Design review of the part built by this model. Coordinates are the model's own, in mm. Give positions to 0.01 mm unless a question says otherwise; leave off trailing zeros. Order: outer loops, then holes, each group sorted by start corner. A loop starts at its lowest first (then second) coordinate and runs counter-clockwise, first axis right, second up. Notation, with made-up numbers: (52.5, 15.25) -> (98.5, 15.25) arc R31 ccw to (98.5, 45.25) -> close; hole circle Ø11 at (-31.75, 81.5). An arc over 180 degrees is marked (long way). Return JSON: item names as keys, results as strings.
```python
from build123d import *

# Parameters (mm, degrees)
SKETCH_1_R      = 1.6
EXTRUDE_1_DEPTH = 2
FILLET_1_R      = 2
FILLET_2_R      = 10
SKETCH_2_R      = 2.5
EXTRUDE_2_DEPTH = 5
SKETCH_3_W      = 23
SKETCH_3_H      = 10
EXTRUDE_4_DEPTH = 5


with BuildPart() as part:
    # 草图1 → 凸台-拉伸1 (new body)
    with BuildSketch(Plane(origin=(0, 0, 0), x_dir=(1, 0, 0), z_dir=(0, 1, 0))):
        Polygon((-11.5, 4.501120792), (11.5, 4.501120792), (11.5, 1.918654762), (40, 1.918654762), (56.146384284, 15.918654762), (90, 15.918654762), (90, 29.918654762), (-90, 29.918654762), (-90, 15.918654762), (-56.146384284, 15.918654762), (-40, 1.918654762), (-11.5, 1.918654762), align=None)
        with Locations(Location((17.5, 7.896444982, 0), (0, 0, 270))):
            Circle(SKETCH_1_R, mode=Mode.SUBTRACT)
        with Locations(Location((25, 7.896444982, 0), (0, 0, 270))):
            Circle(SKETCH_1_R, mode=Mode.SUBTRACT)
        with Locations(Location((32.5, 7.896444982, 0), (0, 0, 270))):
            Circle(SKETCH_1_R, mode=Mode.SUBTRACT)
        with Locations(Location((-32.5, 7.896444982, 0), (0, 0, 90))):
            Circle(SKETCH_1_R, mode=Mode.SUBTRACT)
        with Locations(Location((-25, 7.896444982, 0), (0, 0, 90))):
            Circle(SKETCH_1_R, mode=Mode.SUBTRACT)
        with Locations(Location((-17.5, 7.896444982, 0), (0, 0, 90))):
            Circle(SKETCH_1_R, mode=Mode.SUBTRACT)
    extrude(amount=EXTRUDE_1_DEPTH)

    # 圆角1
    fillet_1_edges = [part.edges().sort_by_distance(p)[0] for p in [
        (-11.5, 1, -1.918654762),
        (-90, 1, -15.918654762),
        (-90, 1, -29.918654762),
        (90, 1, -29.918654762),
        (90, 1, -15.918654762),
        (11.5, 1, -1.918654762),
    ]]
    fillet(fillet_1_edges, radius=FILLET_1_R)

    # 圆角2
    fillet_2_edges = [part.edges().sort_by_distance(p)[0] for p in [
        (-56.146384284, 1, -15.918654762),
        (56.146384284, 1, -15.918654762),
    ]]
    fillet(fillet_2_edges, radius=FILLET_2_R)

    # 草图2 → 凸台-拉伸2 (add)
    with BuildSketch(Plane.XZ):
        with Locations(Location((-8, -22.918654762, 0), (0, 0, 90))):
            Circle(SKETCH_2_R)
        with Locations(Location((-24, -22.918654762, 0), (0, 0, 90))):
            Circle(SKETCH_2_R)
        with Locations(Location((-40, -22.918654762, 0), (0, 0, 90))):
            Circle(SKETCH_2_R)
        with Locations(Location((-56, -22.918654762, 0), (0, 0, 90))):
            Circle(SKETCH_2_R)
        with Locations(Location((-72, -22.918654762, 0), (0, 0, 90))):
            Circle(SKETCH_2_R)
        with Locations(Location((-86, -22.918654762, 0), (0, 0, 90))):
            Circle(SKETCH_2_R)
        with Locations(Location((8, -22.918654762, 0), (0, 0, 90))):
            Circle(SKETCH_2_R)
        with Locations(Location((24, -22.918654762, 0), (0, 0, 90))):
            Circle(SKETCH_2_R)
        with Locations(Location((40, -22.918654762, 0), (0, 0, 90))):
            Circle(SKETCH_2_R)
        with Locations(Location((56, -22.918654762, 0), (0, 0, 90))):
            Circle(SKETCH_2_R)
        with Locations(Location((72, -22.918654762, 0), (0, 0, 90))):
            Circle(SKETCH_2_R)
        with Locations(Location((86, -22.918654762, 0), (0, 0, 90))):
            Circle(SKETCH_2_R)
    extrude(amount=EXTRUDE_2_DEPTH)

    # 草图3 → 凸台-拉伸4 (add)
    with BuildSketch(Plane(origin=(0, 2, 0), x_dir=(1, 0, 0), z_dir=(0, 1, 0))):
        with Locations((0, 9.501120792)):
            Rectangle(SKETCH_3_W, SKETCH_3_H)
    extrude(amount=EXTRUDE_4_DEPTH)


solid = part.part
```
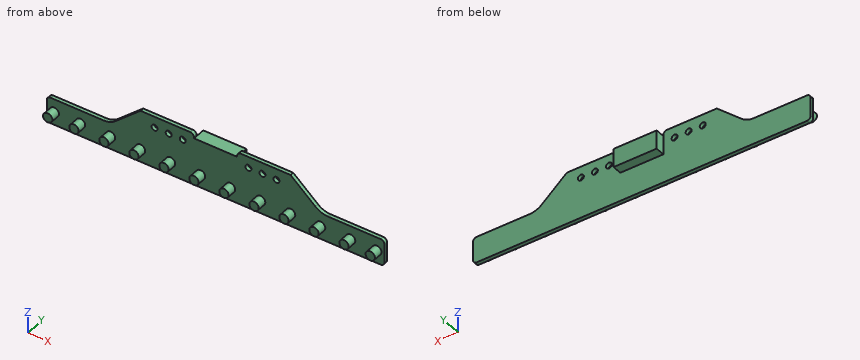
Item 1: Add section B-B (x = 72). Give the boundary of the cut face in (y, z).
Result set:
{"outline": "(-5, -25.42) -> (0, -25.42) -> (0, -29.92) -> (2, -29.92) -> (2, -15.92) -> (0, -15.92) -> (0, -20.42) -> (-5, -20.42) -> close"}
Item 2: Wall thickness on L1, parallel to Z at x = -17.5, y = 0.55; L2, parallel to Y at x = 46, z = -11.25; L3, parallel to X at y = 4.25, z = -7.25: over which ranges is each line inside the solid? List them lowest first. Write a range as [from, to].
Result set:
{"L1": "z = [-29.92, -9.5], [-6.3, -1.92]", "L2": "y = [0, 2]", "L3": "x = [-11.5, 11.5]"}
Item 3: Add section C-C (y = 3.75). Give the boundary of the cut face in (x, z).
Result set:
{"outline": "(-11.5, -14.5) -> (11.5, -14.5) -> (11.5, -4.5) -> (-11.5, -4.5) -> close"}
Item 4: For pin 1 (10 mm diameter, centred on x = 41.5, z = -12.5, fed in from -Y); pin 2 (1.9 mm diameter, centred on x = -32.5, z = -7.9, fed in from +Y); pin 3 (3 mm diameter, centred on x = -5, z = -24.5, fed in from +Y); pin 4 (1.6 mm diameter, centred on x = -74.5, y = 0.5, fed in from +Z), all flat-tipped, find the tip position at first contact; note any pin that passes through.
Result set:
{"pin 1": "stops at y = 0", "pin 2": "passes through", "pin 3": "stops at y = 2", "pin 4": "stops at z = -15.92"}
Item 5: Add section A-A (x = 32.5). Give the boundary of the cut face in (y, z), plus the area to 3 significant figures.
Result set:
{"outline": "(0, -29.92) -> (2, -29.92) -> (2, -9.5) -> (0, -9.5) -> close; (0, -6.3) -> (2, -6.3) -> (2, -1.92) -> (0, -1.92) -> close", "area": "49.6 mm^2"}
